from build123d import *

# Parameters (mm, degrees)
F1_DEPTH = 19.05
F3_D     = 5.1054
F4_SIZE  = 5.08
F6_DEPTH = 25.4
F8_D     = 7.9375
F8_DEPTH = 17.4752
F8_TIP   = 2.3846655818


with BuildPart() as f1:
    # F0 (on Top) → F1 (new body)
    with BuildSketch(Plane.XY):
        with BuildLine():
            Line((0, 50.8), (0, 0))
            Line((0, 0), (15.875, 0))
            ThreePointArc((15.875, 0), (31.75, 15.875), (47.625, 0))
            Line((47.625, 0), (63.5, 0))
            Line((63.5, 0), (63.5, 50.8))
            Line((63.5, 50.8), (0, 50.8))
        make_face()
    extrude(amount=F1_DEPTH)

    # F3 (through all)
    with Locations(Plane(origin=(0, 50.8, 0), x_dir=(-1, 0, 0), z_dir=(0, 1, 0))):
        with Locations((-55.5625, 9.525), (-7.9375, 9.525)):
            Hole(F3_D / 2)

    # F4
    f4_edges = [f1.edges().sort_by_distance(p)[0] for p in [
        (63.5, 50.8, 9.525),
        (0, 50.8, 9.525),
    ]]
    chamfer(f4_edges, length=F4_SIZE)

    # F5 (on face) → F6 (cut)
    with BuildSketch(Plane.XY.offset(19.05)):
        with BuildLine():
            Line((0, 3.175), (0, 0))
            Line((0, 0), (15.875, 0))
            ThreePointArc((15.875, 0), (15.955388571, 1.5955797718), (16.1957401333, 3.175))
            Line((16.1957401333, 3.175), (0, 3.175))
        make_face()
        with BuildLine():
            ThreePointArc((47.3042598667, 3.175), (47.544611429, 1.5955797718), (47.625, 0))
            Line((47.625, 0), (63.5, 0))
            Line((63.5, 0), (63.5, 3.175))
            Line((63.5, 3.175), (47.3042598667, 3.175))
        make_face()
    extrude(amount=-F6_DEPTH, mode=Mode.SUBTRACT)

    # F8
    with Locations(Plane(origin=(0, 50.8, 0), x_dir=(-1, 0, 0), z_dir=(0, 1, 0))):
        with Locations((-31.75, 9.525)):
            Hole(F8_D / 2, depth=F8_DEPTH)
            with Locations((0, 0, -(F8_DEPTH + F8_TIP / 2))):  # 118° drill point
                Cone(0, F8_D / 2, F8_TIP, mode=Mode.SUBTRACT)


solid = f1.part
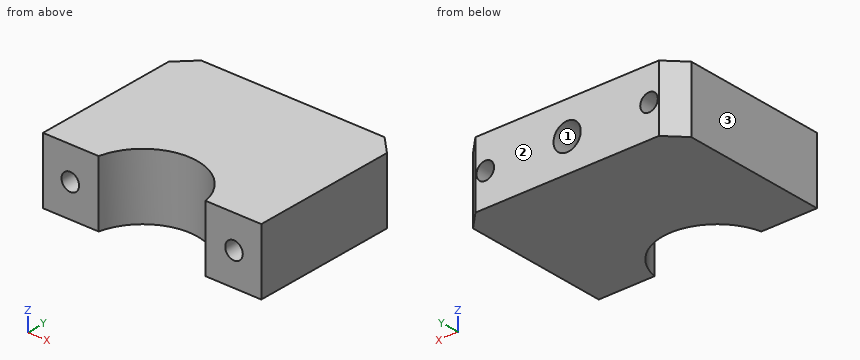
Design review of the part built by this model. Coordinates are the model's own, in mm. Face numbers are marked on the shaded views. Give positions to 0.01 mm unless a question says otherwise; leave off trailing zeros. Write each loop counter-clockwise with the first axis right and the second up, starting at its lowest first coordinate (ties: lowest second). Pieces come first, ordered by that corner, then holes. Notation, with made-up numbers: M 27.5,11 L 40.5,11 A16 cw 40.5,41 Z; hole C 0,44.25 d3. An arc over 180 degrees is marked long. Return JSON: item names as keys, results as strings. Group by question number.
Item 1: Clearance check with flat-ended pins moving along their axes: pin 1 Ø7 at (x, z) = (31.75, 9.525) entering from -Y; pin 2 Ø6 at (x, z) = (43, 15.5) entering from -Y; pin 3 Ø2 at (x, z) = (19, 5) entering from -Y. State where each tip first meets the part, or that it passes through.
Item 2: Take a section at B-B (z = 15.5). Give the boundary of the cut face in (x, y) (3 decimals).
Item 3: Wall thickness on line 1 along X through (y, z) = (34, 9.75); line 2 along X through (y, z) = (33.5, 8.5); line 3 along Z through (x, y) = (55.5, 45): over which ranges is each line inside the solid? List them lowest first.
Item 4: The part is to be moulded in two halves that separate along X. For the marked faces 1, 2 and 3, say which applies: pulls with the +X half, pulls with the -X half, needs draft (parallel to the pull), parting line crosses it, or undercut.
Item 5: Take a section at A-A (y = 8.5). Count the separate pieces of the cut face and the enclosed holes in it, plus the area to 3 significant figures.
Return value:
{
 "1": {"pin 1": "stops at y = 15.48", "pin 2": "stops at y = 7", "pin 3": "stops at y = 7.93"},
 "2": {"outline": "M 0,3.175 L 16.196,3.175 A15.875 cw 47.304,3.175 L 63.5,3.175 L 63.5,45.72 L 58.42,50.8 L 5.08,50.8 L 0,45.72 Z"},
 "3": {"line 1": "x = 0 to 5.39, 10.48 to 27.79, 35.71 to 53.02, 58.11 to 63.5", "line 2": "x = 0 to 5.6, 10.28 to 27.92, 35.58 to 53.22, 57.9 to 63.5", "line 3": "z = 0 to 6.97, 12.08 to 19.05"},
 "4": {"face 1": "undercut", "face 2": "needs draft", "face 3": "pulls with the -X half"},
 "5": {"separate pieces": "2", "enclosed holes": "2", "area": "658 mm2"}
}
